Part model, mm, in its own coordinate system. Face numbers are marked on the shaded views. A direction names the side the tool comes from. Give positions to 0.01 mm unless a question says otherwise; leave off trailing zeros. Write each loop counter-clockwise with the first axis right and the second up, starting at its lowest first coordinate (ties: lowest second). Pieces come first, ordered by that corner, then holes.
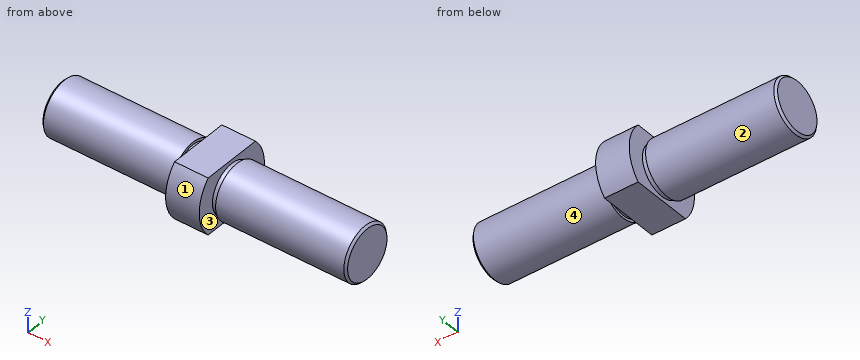
```python
from build123d import *

# Parameters (mm, degrees)
EXTRUDE_1_DEPTH = 13
SKETCH_2_R      = 19
EXTRUDE_2_DEPTH = 105
SKETCH_3_R      = 21
EXTRUDE_3_DEPTH = 101
CHAMFER_1_SIZE  = 1.648


with BuildPart() as part:
    # Эскиз1 → Бобышка-Вытянуть1 (new body)
    with BuildSketch(Plane(origin=(0, 0, 0), x_dir=(0, 0, -1), z_dir=(1, 0, 0))):
        with BuildLine():
            Line((22, -23.237900077), (22, 23.237900077))
            ThreePointArc((22, 23.237900077), (0, 32), (-22, 23.237900077))
            Line((-22, 23.237900077), (-22, -23.237900077))
            ThreePointArc((-22, -23.237900077), (0, -32), (22, -23.237900077))
        make_face()
    extrude(amount=EXTRUDE_1_DEPTH)

    # Эскиз2 → Бобышка-Вытянуть2 (add)
    with BuildSketch(Plane(origin=(13, 0, 0), x_dir=(0, 0, -1), z_dir=(1, 0, 0))):
        Circle(SKETCH_2_R)
    extrude(amount=EXTRUDE_2_DEPTH)

    # Эскиз3 → Бобышка-Вытянуть3 (add)
    with BuildSketch(Plane(origin=(118, 0, 0), x_dir=(0, 0, -1), z_dir=(1, 0, 0))):
        Circle(SKETCH_3_R)
    extrude(amount=-EXTRUDE_3_DEPTH)

    # Фаска1
    chamfer_1_edges = [part.edges().sort_by_distance(p)[0] for p in [
        (118, 0, 21),
    ]]
    chamfer(chamfer_1_edges, length=CHAMFER_1_SIZE)

    # Зеркальное отражение4: part across plane


with BuildPart() as part_1:
    add(part.part)
    add(part.part.mirror(Plane(origin=(0, 0, 0), x_dir=(0, 0, 1), z_dir=(1, 0, 0))))


solid = part_1.part
```
1) 3-axis set-ups, long thin cutter, end or side, ignore diameter. For the marked faces 1, 2, 3 and 4: which of +Z, -Z, +X, -X, +Y, -Y reach the whole face in a straight line?
Answers follow:
face 1: +X, -X, -Y
face 2: -X
face 3: none
face 4: +X
2) Wall check: L1, parallel to Y at x = -51.5, z = 9; L2, parallel to Y at x = 26, z = -1; L3, parallel to Z at x = -72.5, y = 18.5. Give the ranges that are in metal, low to high.
Answers follow:
L1: y = -18.97 to 18.97
L2: y = -20.98 to 20.98
L3: z = -9.94 to 9.94
3) Saw through at A-A, the plane z = 0. Write the cut outline in (x, y), then the cut area to 3 significant figures.
Answers follow:
outline: (-118, -19.35) - (-116.35, -21) - (-17, -21) - (-17, -19) - (-13, -19) - (-13, -32) - (13, -32) - (13, -19) - (17, -19) - (17, -21) - (116.35, -21) - (118, -19.35) - (118, 19.35) - (116.35, 21) - (17, 21) - (17, 19) - (13, 19) - (13, 32) - (-13, 32) - (-13, 19) - (-17, 19) - (-17, 21) - (-116.35, 21) - (-118, 19.35) - close
area: 10,400 mm2
4) Saw through at B-B, the plane y = 0. Write the cut outline in (x, z).
Answers follow:
outline: (-118, -19.35) - (-116.35, -21) - (-17, -21) - (-17, -19) - (-13, -19) - (-13, -22) - (13, -22) - (13, -19) - (17, -19) - (17, -21) - (116.35, -21) - (118, -19.35) - (118, 19.35) - (116.35, 21) - (17, 21) - (17, 19) - (13, 19) - (13, 22) - (-13, 22) - (-13, 19) - (-17, 19) - (-17, 21) - (-116.35, 21) - (-118, 19.35) - close
5) Saw through at C-C, the plane x = -49. Write the cut outline in (y, z), then the cut area to 3 significant figures.
Answers follow:
outline: circle Ø42 at (0, 0)
area: 1,390 mm2
6) Saw through at D-D, the plane x = 8. Write the cut outline in (y, z), then the cut area to 3 significant figures.
Answers follow:
outline: (-23.24, -22) - (23.24, -22) arc R32 ccw to (23.24, 22) - (-23.24, 22) arc R32 ccw to start
area: 2,570 mm2
7) Pin check, flat tips, straight feed: pin 1 Ø10 at (x, z) = (-49, -4.5) entering from -Y; pin 2 Ø1 at (x, y) = (87.5, -4) entering from +Z; pin 3 Ø2 at (x, z) = (66, 7) entering from -Y. Stop position of each tip, or through.
Answers follow:
pin 1: stops at y = -21
pin 2: stops at z = 20.71
pin 3: stops at y = -20.12
